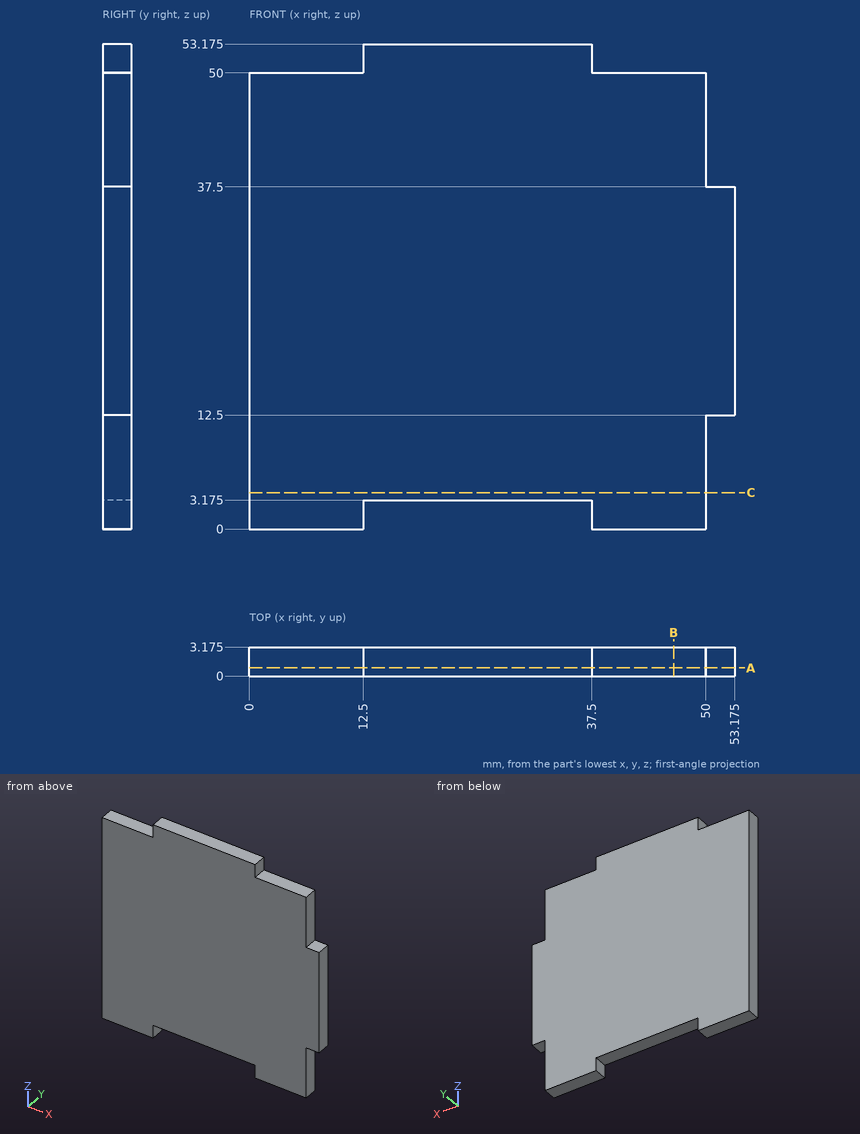
Can you work these out from the drawing? Everything is in mm from the part's minimum corner. Coordinates: 2 decimals unless noted, no trailing zeros. Write each loop counter-clockwise with the first axis right and the second up, starting at its lowest first coordinate (ties: lowest second). Pieces come first, ordered by that corner, then holes. Notation, with made-up numbers: (-27, 42.5) -> (27, 42.5) arc R15 cw to (27, 47.5) -> close; hole circle Ø4 at (-32, 3). An arc over 180 degrees is marked (long way). Return JSON: item names as keys, results as strings.
(1) Imagine slicing it at A-A, the plane y = 0.9. Please give me the cut outline in (x, z) (3 decimals).
Numbers:
{"outline": "(0, 0) -> (12.5, 0) -> (12.5, 3.175) -> (37.5, 3.175) -> (37.5, 0) -> (50, 0) -> (50, 12.5) -> (53.175, 12.5) -> (53.175, 37.5) -> (50, 37.5) -> (50, 50) -> (37.5, 50) -> (37.5, 53.175) -> (12.5, 53.175) -> (12.5, 50) -> (0, 50) -> close"}
(2) I need wall thicknesses on L1, parallel to Z at x = 20, y = 1.05 (3 decimals); L2, parallel to X at y = 1.95, z = 38.5; L3, parallel to X at y = 2.6, z = 51. Which ranges of each line are inside material? Lowest first, please.
Numbers:
{"L1": "z = 3.175 to 53.175", "L2": "x = 0 to 50", "L3": "x = 12.5 to 37.5"}
(3) Imagine slicing it at B-B, the plane x = 46.5. Please give me the cut outline in (y, z) (3 decimals), then the cut area to 3 significant figures.
Numbers:
{"outline": "(0, 0) -> (3.175, 0) -> (3.175, 50) -> (0, 50) -> close", "area": "159 mm2"}
(4) Imagine slicing it at C-C, the plane z = 4. Please give me the cut outline in (x, y) (3 decimals), then the cut area to 3 significant figures.
Numbers:
{"outline": "(0, 0) -> (50, 0) -> (50, 3.175) -> (0, 3.175) -> close", "area": "159 mm2"}
(5) I'm going to push flat-ended pins straight in: pin 1 (1 mm diameter, centred on y = 2, z = 42.5, fed in from +X); pin 2 (1.6 mm diameter, centred on x = 31, y = 2.5, fed in from -Z) (3 decimals); pin 3 (1 mm diameter, centred on x = 7.5, y = 2.5, fed in from +Z). Where does each tip first touch, or does it pass through?
Numbers:
{"pin 1": "stops at x = 50", "pin 2": "stops at z = 3.175", "pin 3": "stops at z = 50"}
